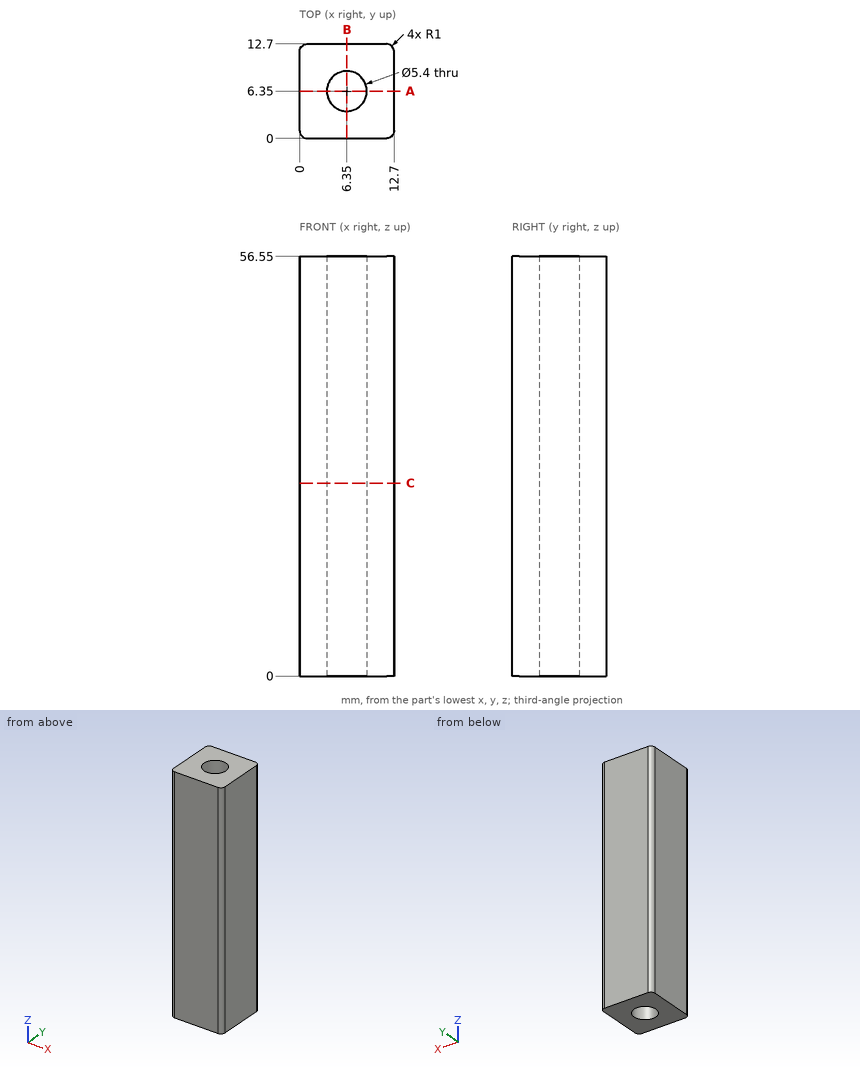
Here's the drawing with two shaded views (mm, measured from the low corner). I have some questions. Round coordinates to 2 decimals unless told otherwise and drop trailing zeros. Write each loop counter-clockwise with the first axis right and the second up, starting at its lowest first coordinate (ties: lowest second). Pieces come first, ordered by that corner, then holes. Notation, with made-up numbers: M 42.5,-15 L 90.5,-15 A15 ccw 90.5,-2 Z; hole C 87,12.5 d5. An arc over 180 degrees is marked long. Answer in a Markdown table with one row per item. Add a question column.
Q1. Imagine slicing it at C-C (z = 26). Please give me the cut outline in (x, y).
Q2. If I drill on line 1 (X direction, y = 6.5, z = 52.5); line 2 (X direction, y = 8.5, z = 35), over which ranges is the centre line in solid material (lowest first)? Write a range as from..to.
Q3. Imagine slicing it at A-A (y = 6.35). Please give me the cut outline in (x, z), then the cut area to 3 significant figures.
Values:
| question | item | result |
|---|---|---|
| 1 | outline | M 0,1 A1 ccw 1,0 L 11.7,0 A1 ccw 12.7,1 L 12.7,11.7 A1 ccw 11.7,12.7 L 1,12.7 A1 ccw 0,11.7 Z; hole C 6.35,6.35 d5.4 |
| 2 | line 1 | 0..3.65, 9.05..12.7 |
| 2 | line 2 | 0..4.72, 7.98..12.7 |
| 3 | outline | M 0,0 L 3.65,0 L 3.65,56.55 L 0,56.55 Z; M 9.05,0 L 12.7,0 L 12.7,56.55 L 9.05,56.55 Z |
| 3 | area | 413 mm^2 |
